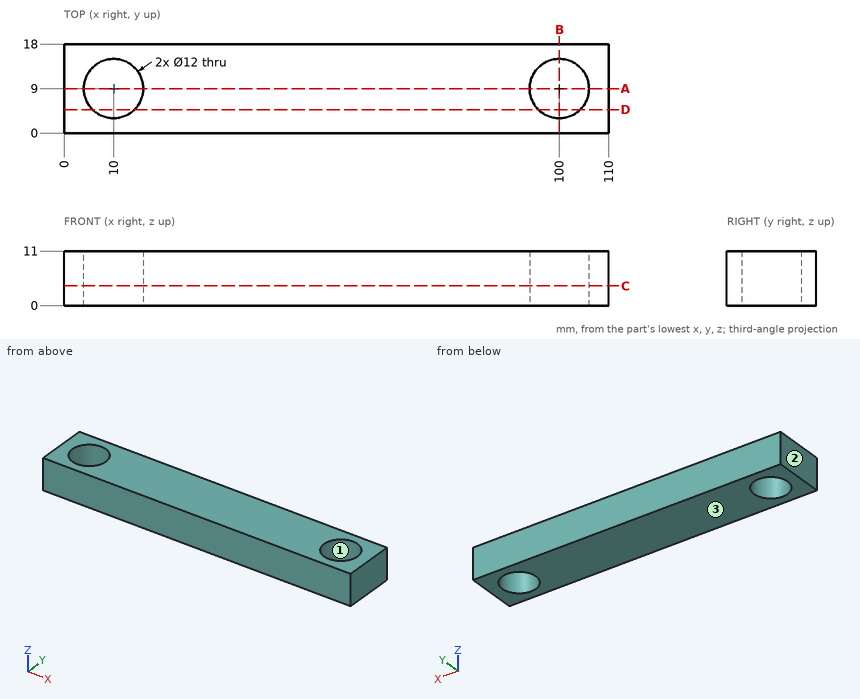
Geometry check sheet. Reference: drawing and pictorial views, mm from the part's lowest x, y, z. Round coordinates to 2 decimals unless told otherwise and drop trailing zeros. Write each loop counter-clockwise with the first axis right and the second up, starting at its lowest first coordinate (ties: lowest second). Pieces come first, ordered by that corner, then holes.
1. Section check B-B on x = 100. Enter the section's corners in (y, z), plus the area to 3 significant figures.
2. Draft check along X on the marked faces 1, 2 and 3. Enter one of: +X half, -X half, draft (parallel to the pull), parting line (faces both ways), or undercut.
3. Section check A-A on y = 9. Enter the section's corners in (x, z), plus the area to 3 significant figures.
4. Section check D-D on y = 4.75. Enter the section's corners in (x, z).
5. Scan lines: L1, parallel to X at y = 9, z = 4.5; L2, parallel to Y at x = 100, z = 4.75; L3, parallel to X at y = 11, z = 2.5. Record each from-to range of solid material in increasing order.
6. Section check C-C on z = 4. Enter the section's corners in (x, y).
Answer:
1. outline: (0, 0) - (3, 0) - (3, 11) - (0, 11) - close; (15, 0) - (18, 0) - (18, 11) - (15, 11) - close
1. area: 66.0 mm2
2. face 1: undercut
2. face 2: -X half
2. face 3: draft
3. outline: (0, 0) - (4, 0) - (4, 11) - (0, 11) - close; (16, 0) - (94, 0) - (94, 11) - (16, 11) - close; (106, 0) - (110, 0) - (110, 11) - (106, 11) - close
3. area: 946 mm2
4. outline: (0, 0) - (5.76, 0) - (5.76, 11) - (0, 11) - close; (14.24, 0) - (95.76, 0) - (95.76, 11) - (14.24, 11) - close; (104.24, 0) - (110, 0) - (110, 11) - (104.24, 11) - close
5. L1: x = 0 to 4, 16 to 94, 106 to 110
5. L2: y = 0 to 3, 15 to 18
5. L3: x = 0 to 4.34, 15.66 to 94.34, 105.66 to 110
6. outline: (0, 0) - (110, 0) - (110, 18) - (0, 18) - close; hole circle Ø12 at (10, 9); hole circle Ø12 at (100, 9)
